```python
from build123d import *

# Parameters (mm, degrees)
F0_W     = 76.2
F0_H     = 50.8
F2_DEPTH = 4.826
F3_W     = 76.2
F3_H     = 38.1
F4_DEPTH = 3.81
F5_W     = 76.2
F5_H     = 12.7
F6_DEPTH = 3.81


with BuildPart() as f2:
    # F0 (on Top) → F2 (new body)
    with BuildSketch(Plane.XY):
        Rectangle(F0_W, F0_H)
    extrude(amount=F2_DEPTH)

    # F3 (on face) → F4 (join)
    with BuildSketch(Plane.XZ.offset(25.4)):
        with Locations((0, 19.05)):
            Rectangle(F3_W, F3_H)
    extrude(amount=F4_DEPTH)

    # F5 (on face) → F6 (join)
    with BuildSketch(Plane(origin=(0, 25.4, 0), x_dir=(-1, 0, 0), z_dir=(0, 1, 0))):
        with Locations((0, 6.35)):
            Rectangle(F5_W, F5_H)
    extrude(amount=F6_DEPTH)


solid = f2.part
```
Source: CAD feature listing. Evaluate the final solid. Frame: model axes, mm. A direction names the side the tool comes from. Round coordinates to 2 decimals unless told otherwise and drop trailing zeros. Loops run counter-clockwise (first coordinate to the right, second up) from the corner with the lowest first, then second, coordinate; pieces in that order, holes last. Notation, with made-up numbers: (-23.5, 24.25) - (35.5, 24.25) arc R24 cw to (35.5, 53.25) - close; hole circle Ø10 at (29.25, 19.5). An arc over 180 degrees is marked (long way). Use CSV: the item, a comma, the result in double quotes.
Q1. Reachability of faces 1 (the flat face through (1, 0, 0)), 2 (the flat face through (-1, -25.4, 22)) from +Z, -Z, +X, -X, +Y, -Y: full face, straight path, thin tool, end or side. Return the list, or none.
Reported:
face 1,"-Z, +X, -X, +Y, -Y"
face 2,"+Z, +X, -X"
Q2. Ray query, line 1 along Y through (x, z) = (29.5, 6); line 2 along Y through (x, z) = (-10.5, 13.5); line 3 along Z through (x, y) = (23, 16). Return the intervals inside material, ascending.
Reported:
line 1,"-29.21 to -25.4, 25.4 to 29.21"
line 2,"-29.21 to -25.4"
line 3,"0 to 4.83"
Q3. Section query A-A, the plane z = 7. Output: boundary loops of the cut face in (x, y), then the cut area to 3 significant figures.
Reported:
outline,"(-38.1, -29.21) - (38.1, -29.21) - (38.1, -25.4) - (-38.1, -25.4) - close; (-38.1, 25.4) - (38.1, 25.4) - (38.1, 29.21) - (-38.1, 29.21) - close"
area,"581 mm^2"
Q4. Section query D-D, the plane y = 0. Output: boundary loops of the cut face in (x, z), then the cut area to 3 significant figures.
Reported:
outline,"(-38.1, 0) - (38.1, 0) - (38.1, 4.83) - (-38.1, 4.83) - close"
area,"368 mm^2"
Q5. Pin query (flat end, axial travel): pin 1 Ø12 at (x, y) = (28.5, 9) entering from +Z; pin 2 Ø12 at (x, z) = (-3.5, 25.5) entering from +Y; pin 3 Ø3 at (x, y) = (14.5, 27.5) entering from +Z. Return the tip coordinate at first contact, or that it passes through.
Reported:
pin 1,"z = 4.83"
pin 2,"y = -25.4"
pin 3,"z = 12.7"
Q6. Section query C-C, the plane z = 32.5. Output: boundary loops of the cut face in (x, y).
Reported:
outline,"(-38.1, -29.21) - (38.1, -29.21) - (38.1, -25.4) - (-38.1, -25.4) - close"
Q7. Section query B-B, the plane x = -24.5. Output: boundary loops of the cut face in (y, z), then the cut area to 3 significant figures.
Reported:
outline,"(-29.21, 0) - (29.21, 0) - (29.21, 12.7) - (25.4, 12.7) - (25.4, 4.83) - (-25.4, 4.83) - (-25.4, 38.1) - (-29.21, 38.1) - close"
area,"439 mm^2"
Q8. Mould query, pull axis Y, two halves, no side actions, for faces 3 (the flat face through (1, 25.4, 9)), 4 (the flat face through (-1, -29.21, 19)), 5 (the flat face through (1, 27, 12.7)). Classes: pulls with the +Y half, pulls with the -Y half, needs draft (parallel to the pull), parting line crosses it, or undercut.
Reported:
face 3,"undercut"
face 4,"pulls with the -Y half"
face 5,"needs draft"
